Check sheet for the modelled part. Datum: model origin and axes. Units: mm. A direction names the side the tool comes from. Round coordinates to 2 decimals unless told otherwise and drop trailing zeros. Order: outer loops, then holes, each group sorted by start corner. A loop starts at its lowest first (then second) coordinate and runs counter-clockwise, first axis right, second up.
Q1. Cross-section at B-B on y = 10. Record the cut outline in (x, z).
Q2. Cross-section at A-A on x = 5. Record the cut outline in (y, z).
Q3. Cross-section at D-D on y = 71.5. Record the cut outline in (x, z), then the cut area to 3 significant figures.
Q4. Scan lines: probe 1 along X at (y, z) = (80.25, 0); probe 2 along Y at (x, z) = (5.5, 0); probe 3 along Z at (x, y) = (5, 10). Record each from-to range of solid material in increasing order.
Q5. Depth check by flat-ended pin: P1, Ø12, axis at y = 15, z = -3, coming from the -X side; P2, Ø0.8, axis at x = 11, z = -1, coming from the -Y side; P3, Ø11.5, axis at y = 10, z = 0, coming from the +X side; P4, Ø8, axis at x = 10.5, z = -6, coming from the -Y side. Enter the tip coordinate at first touch or a pass-through.
Q6. Cross-section at C-C on z = 0. Record the cut outline in (x, y), then the cut area to 3 significant figures.
Q7. Set-up check for faces 4 (the flat face through (10, 37, 0)), 5 (the flat face through (5, 67, 0)), 6 (the flat face through (0, 39, 0)), 7 (the flat face through (5, 44, 10)): record each of +Z, -Z, +X, -X, +Y, -Y from which the full face is reachable in a straight line by a thin tool's end or side.
Q8. Mould release check, pull along Y, two halves, no side actions. Record for faces 1 (the cylindrical face through (5.07, 5.043, -0.651)), 2 (the cylindrical face through (2.6, 76.1, 1.8)), 3 (the cylindrical face through (5.06, 0.57, -9.4)): +Y half, -Y half, draft (parallel to the pull), parting line (faces both ways), or undercut.
Autodesk Inventor part; units mm, degrees
ref_plane "YZ Plane" through (0, 0, 0) normal (1, 0, 0) x (0, 1, 0)
ref_plane "XZ Plane" through (0, 0, 0) normal (0, 1, 0) x (-1, 0, 0)
ref_plane "XY Plane" through (0, 0, 0) normal (0, 0, 1) x (1, 0, 0)
sketch "Sketch1" plane through (0, 0, 0) normal (0, 0, 1) x (1, 0, 0)
  line L0 (0, 0) -> (10, 0)
  line L1 (10, 0) -> (10, 85)
  line L2 (10, 85) -> (0, 85)
  line L3 (0, 85) -> (0, 0)
  dimension "d0" = 10
  dimension "d1" = 85
extrude "Extrusion1" add sketch "Sketch1" along normal mid plane 20
sketch "Sketch2" plane through (0, 0, 10) normal (-1, 0, 0) x (0, 0, 1)
  line L0 (-20, 0) -> (-20, 85)
  line L1 (-20, 0) -> (0, 0)
  line L2 (0, 85) -> (0, 0)
  point P0 (-10, 0)
  point P1 (-10, 10)
  point P2 (-10, 0)
  dimension "d14" = 10
  dimension "d15" = 10
hole "Hole1" at (0, 10, 0) direction (1, 0, 0) diameter 10 end through all
fillet "Fillet1" radius 2 2 edges at (5, 0, -10) (5, 0, 10)
sketch "Sketch4" plane through (0, 0, 0) normal (0, 0, 1) x (1, 0, 0)
  line L0 (-2.5, 85) -> (12.5, 85)
  line L1 (12.5, 85) -> (12.5, 75)
  line L2 (12.5, 75) -> (-2.5, 75)
  line L3 (-2.5, 75) -> (-2.5, 85)
  line L4 (10, 85) -> (0, 85)
  point P0 (0, 0)
  point P1 (5, 85)
  point P2 (5, 85)
  dimension "d27" = 15
  dimension "d28" = 10
  dimension "d29" = 7.5
  dimension "d32" = 0
extrude "Extrusion3" add sketch "Sketch4" along normal mid plane 20
sketch "Sketch3" plane through (0, 85, 10) normal (0, 1, 0) x (1, 0, 0)
  circle A0 centre (5, 10) radius 3
  point P0 (0, 10)
  dimension "d24" = 6
extrude "Extrusion2" cut sketch "Sketch3" along normal blind 20 and the other way blind 18
fillet "Fillet2" radius 1 2 edges at (-2.5, 75, 0) (12.5, 75, 0)
fillet "Fillet3" radius 1 22 edges at (10, 0.5858, 9.4142) (10, 0, 0) (10, 0.5858, -9.4142) (10, 38.5, -10) (10, 38.5, 10) (0, 0.5858, 9.4142) (0, 0, 0) (0, 0.5858, -9.4142) (0, 38.5, -10) (0, 38.5, 10) (-0.75, 75, 10) (-2.5, 80.5, 10) (12.5, 85, 0) (-2.5, 85, 0) (5, 85, 10) (5, 85, -10) (10.75, 75, -10) (12.5, 80.5, -10) (10.75, 75, 10) (12.5, 80.5, 10) (-0.75, 75, -10) (-2.5, 80.5, -10)
properties part number "Suporte da base movel"
Results found:
1. outline: (0, -9) arc R1 ccw to (1, -10) - (9, -10) arc R1 ccw to (10, -9) - (10, -5) - (0, -5) - close; (0, 5) - (10, 5) - (10, 9) arc R1 ccw to (9, 10) - (1, 10) arc R1 ccw to (0, 9) - close
2. outline: (0, -8) arc R2 ccw to (2, -10) - (84, -10) arc R1 ccw to (85, -9) - (85, -3) - (67, -3) - (67, 3) - (85, 3) - (85, 9) arc R1 ccw to (84, 10) - (2, 10) arc R2 ccw to (0, 8) - close; hole circle Ø10 at (10, 0)
3. outline: (0, -9) arc R1 ccw to (1, -10) - (9, -10) arc R1 ccw to (10, -9) - (10, 9) arc R1 ccw to (9, 10) - (1, 10) arc R1 ccw to (0, 9) - close; hole circle Ø6 at (5, 0)
3. area: 171 mm2
4. probe 1: x = -2.5 to 2, 8 to 12.5
4. probe 2: y = 0 to 5, 15 to 67
4. probe 3: z = -10 to -5, 5 to 10
5. P1: stops at x = 0
5. P2: stops at y = 75
5. P3: stops at x = 10
5. P4: stops at y = 0
6. outline: (-2.5, 76) arc R1 ccw to (-1.5, 75) - (0, 75) - (0, 15) - (10, 15) - (10, 75) - (11.5, 75) arc R1 ccw to (12.5, 76) - (12.5, 84) arc R1 ccw to (11.5, 85) - (8, 85) - (8, 67) - (2, 67) - (2, 85) - (-1.5, 85) arc R1 ccw to (-2.5, 84) - close; (0, 1) arc R1 ccw to (1, 0) - (9, 0) arc R1 ccw to (10, 1) - (10, 5) - (0, 5) - close
6. area: 691 mm2
7. face 4: +Z, -Z, +X, -Y
7. face 5: +Y
7. face 6: +Z, -Z, -X, -Y
7. face 7: +Z, +X, -X, +Y, -Y
8. face 1: undercut
8. face 2: draft
8. face 3: -Y half
